The listing builds one solid part. Answer for the finished solid, in the listing's coordinates (mm). Face numbers are marked on the shaded views. A direction names the side the tool comes from. Round coordinates to 2 decimals unless told otherwise and drop trailing zeros. Write each loop counter-clockwise with the first axis right and the second up, starting at its lowest first coordinate (ties: lowest second). Pieces come first, ordered by that corner, then holes.
from build123d import *

# Parameters (mm, degrees)
F1_DEPTH = 4
F2_R     = 1
F3_R     = 3
F5_DEPTH = 0.5


with BuildPart() as f1:
    # F0 (on Top) → F1 (new body)
    with BuildSketch(Plane.XY):
        Polygon((-12.124355653, 7), (-30.1414284285, 7), (-44.8717504895, 7), (-33.124355653, -7), (-12.124355653, -7), (0, -14), (12.124355653, -7), (33.124355653, -7), (44.8717504895, 7), (30.1414284285, 7), (12.124355653, 7), (0, 14), align=None)
        Polygon((4.09, 2.361362601), (4.09, -2.361362601), (0, -4.722725202), (-4.09, -2.361362601), (-4.09, 2.361362601), (0, 4.722725202), align=None, mode=Mode.SUBTRACT)
    extrude(amount=F1_DEPTH)

    # F2
    f2_edges = [f1.edges().sort_by_distance(p)[0] for p in [
        (-44.87175, 7, 2),
        (44.87175, 7, 2),
    ]]
    fillet(f2_edges, radius=F2_R)

    # F3
    f3_edges = [f1.edges().sort_by_distance(p)[0] for p in [
        (-33.124356, -7, 2),
        (-12.124356, -7, 2),
        (12.124356, -7, 2),
        (12.124356, 7, 2),
        (-12.124356, 7, 2),
        (0, -14, 2),
        (0, 14, 2),
        (33.124356, -7, 2),
    ]]
    fillet(f3_edges, radius=F3_R)

    # F4 (on face) → F5 (cut)
    with BuildSketch(Plane.XY.offset(4)):
        Polygon((0, -9.9585481157), (8.624355653, -4.9792740578), (8.624355653, 4.9792740578), (0, 9.9585481157), (-8.624355653, 4.9792740578), (-8.624355653, -4.9792740578), align=None)
        Polygon((4.09, 2.361362601), (4.09, -2.361362601), (0, -4.722725202), (-4.09, -2.361362601), (-4.09, 2.361362601), (0, 4.722725202), align=None, mode=Mode.SUBTRACT)
        Polygon((-12.124355653, 3.5), (-41.9349017803, 3.5), (-40.4664774258, 1.75), (-12.124355653, 1.75), align=None)
        Polygon((-12.124355653, -1.75), (-37.5296287167, -1.75), (-36.0612043621, -3.5), (-12.124355653, -3.5), align=None)
        Polygon((12.124355653, 3.5), (12.124355653, 1.75), (40.4664774258, 1.75), (41.9349017803, 3.5), align=None)
        Polygon((36.0612043621, -3.5), (37.5296287167, -1.75), (12.124355653, -1.75), (12.124355653, -3.5), align=None)
    extrude(amount=-F5_DEPTH, mode=Mode.SUBTRACT)


solid = f1.part
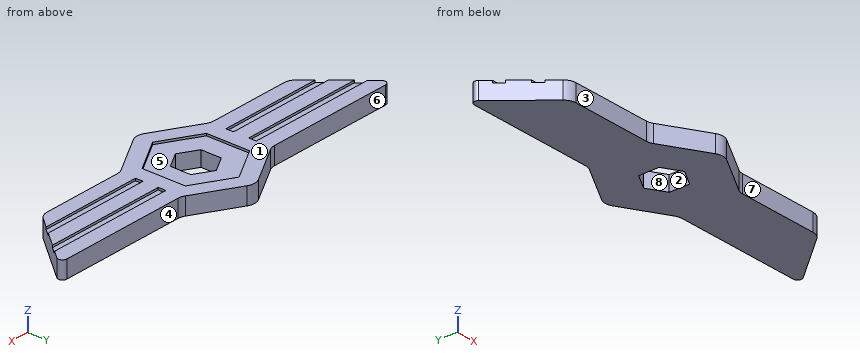
1. Section A-A on z = 1.45 is taken. Determine the outline of the cut face in (x, y), plus the area to 3 significant figures.
Geometry says:
outline: (-43.49, 5.36) - (-34.02, -5.93) arc R3 ccw to (-31.73, -7) - (-12.93, -7) arc R3 cw to (-11.43, -7.4) - (-1.5, -13.13) arc R3 ccw to (1.5, -13.13) - (11.43, -7.4) arc R3 cw to (12.93, -7) - (31.73, -7) arc R3 ccw to (34.02, -5.93) - (43.49, 5.36) arc R1 ccw to (42.73, 7) - (12.93, 7) arc R3 cw to (11.43, 7.4) - (1.5, 13.13) arc R3 ccw to (-1.5, 13.13) - (-11.43, 7.4) arc R3 cw to (-12.93, 7) - (-42.73, 7) arc R1 ccw to start; hole (-4.09, -2.36) - (0, -4.72) - (4.09, -2.36) - (4.09, 2.36) - (0, 4.72) - (-4.09, 2.36) - close
area: 1,200 mm2
2. A tool of negligible diameter and unlimited length cuts with its end or side. For the marked faces 4, 5, 6, 7 and 8, from which of +Z, -Z, +X, -X, +Y, -Y can it reach the whole face along a straight path? Write none if from no direction.
Geometry says:
face 4: +Z, -Z, +X, +Y
face 5: +Z
face 6: +Z, -Z, -X, +Y
face 7: +Z, -Z, +X, -Y
face 8: +Z, -Z
3. Section D-D on x = -16 is taken. Determine the outline of the cut face in (y, z).
Geometry says:
outline: (-7, 0) - (7, 0) - (7, 4) - (3.5, 4) - (3.5, 3.5) - (1.75, 3.5) - (1.75, 4) - (-1.75, 4) - (-1.75, 3.5) - (-3.5, 3.5) - (-3.5, 4) - (-7, 4) - close
4. Given pin 1 (5 mm diameter, centred on x = -2.5, y = -1.5, fed in from +Z); pin 2 (12 mm diameter, centred on x = -34.5, y = -10.5, fed in from -Z); pin 3 (0.6 mm diameter, centred on x = -30, z = 4, fed in from +Y); pin 4 (1.2 mm diameter, centred on x = -21.5, z = 2.5, fed in from -Y), each flat-ended and moving along its own axis, determine where each tip first touches the part or whether it passes through.
Geometry says:
pin 1: stops at z = 3.5
pin 2: stops at z = 0
pin 3: stops at y = 7
pin 4: stops at y = -7
5. Section B-B on x = -3 is taken. Determine the outline of the cut face in (y, z), plus the area to 3 significant figures.
Geometry says:
outline: (-12.27, 0) - (-2.99, 0) - (-2.99, 3.5) - (-8.23, 3.5) - (-8.23, 4) - (-12.27, 4) - close; (2.99, 0) - (12.27, 0) - (12.27, 4) - (8.23, 4) - (8.23, 3.5) - (2.99, 3.5) - close
area: 69.0 mm2
6. Straight lines are drawn through the part: line 1 along Y through (x, z) = (-15, 3.65); line 2 along X through (y, z) = (-2.25, 0.9); line 3 along Y through (x, z) = (31, 1.05). For each, find the intervals that lie inside material, in ascending order.
Geometry says:
line 1: y = -7 to -3.5, -1.75 to 1.75, 3.5 to 7
line 2: x = -37.11 to -4.09, 4.09 to 37.11
line 3: y = -7 to 7
7. Section C-C on y = 0.25 is taken. Determine the outline of the cut face in (x, z).
Geometry says:
outline: (-39.21, 0) - (-4.09, 0) - (-4.09, 3.5) - (-8.62, 3.5) - (-8.62, 4) - (-39.21, 4) - close; (4.09, 0) - (39.21, 0) - (39.21, 4) - (8.62, 4) - (8.62, 3.5) - (4.09, 3.5) - close
8. For a pull along Y with two mould halves and no side action, classify the marked faces 1, 2 and 3 as released by +Y, released by -Y, zero draft, split by the parting line, or undercut.
Geometry says:
face 1: zero draft
face 2: undercut
face 3: released by -Y
